Autodesk Fusion 360 part; units mm, degrees
sketch "Esboço1" plane through (0, 0, 0) normal (0, 1, 0) x (1, 0, 0)
  line L0 (15.7988, 74.5632) -> (15.7988, 7.8598)
  line L1 (0, 7.8598) -> (0, 74.5632)
  circle A0 centre (7.8994, 6.35) radius 2.108
  circle A1 centre (7.8994, 12.7) radius 2.108
  circle A2 centre (7.8994, 19.05) radius 2.108
  circle A3 centre (7.8994, 25.4) radius 2.108
  line L2 (7.8994, 29.21) -> (7.8994, 31.75)
  arc A4 (15.7988, 74.4838) -> (0, 74.4838) centre (7.8994, 74.5235) ccw
  arc A5 (0, 7.9392) -> (15.7988, 7.9392) centre (7.8994, 7.8995) ccw
  arc A6 (5.3594, 31.75) -> (10.4394, 31.75) centre (7.8994, 31.75) ccw
  arc A7 (10.4394, 76.073) -> (5.3594, 76.073) centre (7.8994, 76.073) ccw
  line L3 (5.3594, 31.75) -> (5.3594, 76.073)
  line L4 (10.4394, 31.75) -> (10.4394, 76.073)
  dimension "d4" = 6.35
  dimension "d5" = 6.35
  dimension "d6" = 6.35
  dimension "d8" = 5.08
  dimension "d11" = 4.216
  dimension "d12" = 4.216
  dimension "d13" = 4.216
  dimension "d14" = 4.216
  dimension "d15" = 6.35
  dimension "d16" = 5.08
extrude "Extrusão1" add sketch "Esboço1" along normal blind 4.7752
chamfer "Chanfro1" distance 0.3 angle 45 12 edges at (15.7988, 4.7752, -41.2115) (7.8994, 4.7752, 0) (0, 4.7752, -41.2115) (7.8994, 4.7752, -82.423) (10.4394, 4.7752, -53.9115) (7.8994, 4.7752, -29.21) (5.3594, 4.7752, -53.9115) (7.8994, 4.7752, -78.613) (5.9341, 4.7752, -26.1623) (5.9341, 4.7752, -19.8123) (5.9341, 4.7752, -13.4623) (5.9341, 4.7752, -7.1123)
The model under review builds one solid part; all positions refer to its coordinate system, in mm. A direction names the side the tool comes from. Round coordinates to 2 decimals unless told otherwise and drop trailing zeros. Loops run counter-clockwise (first coordinate to the right, second up) from the corner with the lowest first, then second, coordinate; pieces in that order, holes last. Notation, with made-up numbers: M 56.25,24 L 93.25,24 A15 cw 93.25,49 Z; hole C 76.25,86.25 d3. An arc over 180 degrees is marked long. Answer as CSV lines item,"result".
1. We need section A-A (z = -42). Give the boundary of the cut face in (x, y), plus the area to 3 significant figures.
Outcome:
outline,"M 0,0 L 5.36,0 L 5.36,4.48 L 5.06,4.78 L 0.3,4.78 L 0,4.48 Z; M 10.44,0 L 15.8,0 L 15.8,4.48 L 15.5,4.78 L 10.74,4.78 L 10.44,4.48 Z"
area,"51.0 mm2"
2. For faces 1 (the face through (7.96, 2.21, -29.21)), 2 (the face through (7.958, 4.594, -78.731)), 3 (the face through (7.73, 4.656, -82.24)), list the 3-axis set-ups (+Z, -Z, +X, -X, +Y, -Y) from which the entire face can be reached by the end or side of a thin tool; tool diameter is ignored.
Outcome:
face 1,"+Y, -Y"
face 2,"+Y"
face 3,"-Z, +Y"
3. Draft analysis for pull direction X (two halves, no side actions). For faces 4 (the face through (11, 4.775, -42)), 5 (the face through (8.069, 4.656, -0.183)), 6 (the face through (7.442, 2.206, -27.458)), state which applies: pulls with the +X half, pulls with the -X half, needs draft (parallel to the pull), parting line crosses it, or undercut.
Outcome:
face 4,"needs draft"
face 5,"parting line crosses it"
face 6,"undercut"
4. We need section C-C (z = -12.7). Give the boundary of the cut face in (x, y).
Outcome:
outline,"M 0,0 L 5.79,0 L 5.79,4.48 L 5.49,4.78 L 0.3,4.78 L 0,4.48 Z; M 10.01,0 L 15.8,0 L 15.8,4.48 L 15.5,4.78 L 10.31,4.78 L 10.01,4.48 Z"
5. We need section D-D (x = 8). Count the separate pieces of the cut face and the enclosed holes in it, plus the area to 3 significant figures.
Outcome:
separate pieces,"6"
enclosed holes,"0"
area,"76.7 mm2"
6. We need section B-B (y = 2.05). Give the boundary of the cut face in (x, z), plus the area to 3 significant figures.
Outcome:
outline,"M 0,-74.56 A7.9 ccw 15.8,-74.56 L 15.8,-7.86 A7.9 ccw 0,-7.86 Z; hole M 5.36,-76.07 A2.54 ccw 10.44,-76.07 L 10.44,-31.75 A2.54 ccw 5.36,-31.75 Z; hole C 7.9,-25.4 d4.22; hole C 7.9,-19.05 d4.22; hole C 7.9,-12.7 d4.22; hole C 7.9,-6.35 d4.22"
area,"947 mm2"
7. Insertion check: pin 1 Ø1.3 at (y, z) = (2, -47.5) entering from -X; pin 2 Ø1.5 at (x, y) = (2, 2) entering from -Z; pin 3 Ø2.5 at (x, z) = (7.9, -25.4) entering from -Y. Each pin has a flat end and moves straight along its axis. Give the tip position at first contact, or say it passes through.
Outcome:
pin 1,"stops at x = 0"
pin 2,"stops at z = -80.51"
pin 3,"passes through"
8. To check wall thickness, follow L1, parallel to Z at x = 8, y = 1.95; L2, parallel to X at y = 3.4, z = -19.05; L3, parallel to X at y = 4, z = -73. State the ranges of each line that lie inside material, in increasing order. Write a range as [from, to].
Outcome:
L1,"z = [-82.42, -78.61], [-29.21, -27.51], [-23.29, -21.16], [-16.94, -14.81], [-10.59, -8.46], [-4.24, 0]"
L2,"x = [0, 5.79], [10.01, 15.8]"
L3,"x = [0, 5.36], [10.44, 15.8]"
